```python
from build123d import *

# Parameters (mm, degrees)
SKETCH1_R               = 3
BOSS_EXTRUDE1_DEPTH     = 37.5
SKETCH2_R               = 4
BOSS_EXTRUDE2_DEPTH     = 3
CUT_EXTRUDE1_DEPTH      = 41.893153461
CUT_EXTRUDE1_DEPTH_BACK = 41.893153461
SKETCH3_R               = 1


with BuildPart() as part:
    # Sketch1 → Boss-Extrude1 (new, symmetric)
    with BuildSketch(Plane.XY):
        Circle(SKETCH1_R)
    extrude(amount=BOSS_EXTRUDE1_DEPTH, both=True)

    # Sketch2 → Boss-Extrude2 (add)
    with BuildSketch(Plane(origin=(0, 0, -37.5), x_dir=(-1, 0, 0), z_dir=(0, 0, -1))):
        Circle(SKETCH2_R)
    extrude(amount=BOSS_EXTRUDE2_DEPTH)

    # Sketch3 → Cut-Extrude1 (cut, two sides: drawn at the far end of the back side and taken through both)
    with BuildSketch(Plane(origin=(0, 0, 0), x_dir=(1, 0, 0), z_dir=(0, 1, 0)).offset(-CUT_EXTRUDE1_DEPTH_BACK)):
        with Locations(Location((0, -36, 0), (0, 0, 270))):
            Circle(SKETCH3_R)
    extrude(amount=CUT_EXTRUDE1_DEPTH + CUT_EXTRUDE1_DEPTH_BACK, mode=Mode.SUBTRACT)


solid = part.part
```
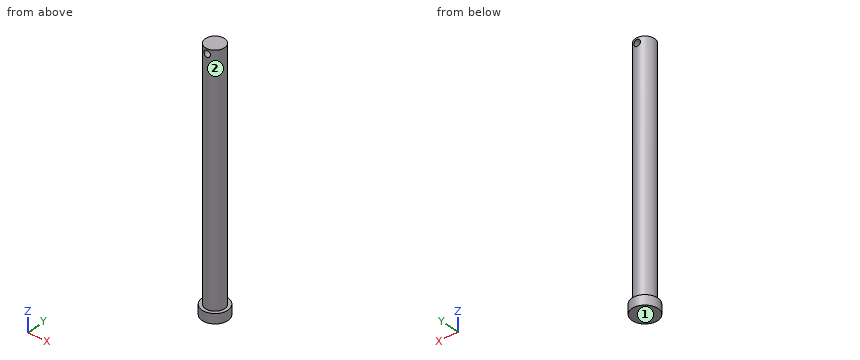
Could you check a few things on this model? Use its own coordinates, in mm. Face numbers are marked on the shaded views. A direction names the side the tool comes from. Give positions to 0.01 mm unless a question says otherwise; leave off trailing zeros. Write each loop counter-clockwise with the first axis right and the second up, starting at its lowest first coordinate (ties: lowest second). Pieces come first, ordered by that corner, then holes. Notation, with made-up numbers: (0, 29.5) - (18, 29.5) arc R19 cw to (18, 62.5) - close; hole circle Ø11 at (68, 13.25). An arc over 180 degrees is marked (long way). One line per item, written item: value. Start each with the question number.
Item 1: Which directions (+Z, -Z, +X, -X, +Y, -Y) give clear straight access to the entire face, cutting with the end or side of a thin tool? Please do the marked faces 1 and 2.
Item 2: Imagine slicing it at A-A, the plane x = 0. List the corners of the cut face in (y, z) for me.
Item 3: Please list where these lines run through material, in increasing order: line 1 (Z direction, x = 0, y = -1); line 2 (X direction, y = 0.25, z = 36); line 3 (Z direction, x = 2, y = 2.75). Write a range as from..to.
Item 4: I'm going to push flat-ended pins straight in: pin 1 (1 mm diameter, centred on y = 0.5, z = 21, fed in from -X); pin 2 (3 mm diameter, centred on x = 0, z = 36, fed in from -Y); pin 3 (1.5 mm diameter, centred on x = -3, y = -2, fed in from +Z). Where does each tip first touch, or does it pass through?
Item 5: Imagine slicing it at C-C, the plane z = -4. List the corners of the cut face in (x, y) for me, and give its area (3 significant figures).
Item 6: Imagine slicing it at B-B, the plane y = 0. List the corners of the cut face in (x, z) for me, and give its area (3 significant figures).
Geometry says:
1. face 1: -Z, +X, -X, +Y, -Y
1. face 2: +Z
2. outline: (-4, -40.5) - (4, -40.5) - (4, -37.5) - (3, -37.5) - (3, 35) - (-3, 35) - (-3, -37.5) - (-4, -37.5) - close; (-3, 37) - (3, 37) - (3, 37.5) - (-3, 37.5) - close
3. line 1: -40.5..35, 37..37.5
3. line 2: -2.99..-1, 1..2.99
3. line 3: -40.5..-37.5
4. pin 1: x = -3
4. pin 2: y = -3
4. pin 3: z = 37.5
5. outline: circle Ø6 at (0, 0)
5. area: 28.3 mm^2
6. outline: (-4, -40.5) - (4, -40.5) - (4, -37.5) - (3, -37.5) - (3, 37.5) - (-3, 37.5) - (-3, -37.5) - (-4, -37.5) - close; hole circle Ø2 at (0, 36)
6. area: 471 mm^2
